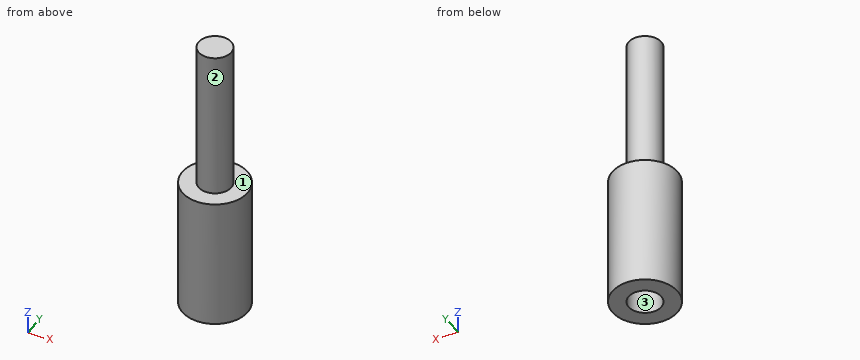
Autodesk Inventor part; units mm, degrees
ref_plane "YZ Plane" through (0, 0, 0) normal (1, 0, 0) x (0, 1, 0)
ref_plane "XZ Plane" through (0, 0, 0) normal (0, 1, 0) x (-1, 0, 0)
ref_plane "XY Plane" through (0, 0, 0) normal (0, 0, 1) x (1, 0, 0)
sketch "Sketch1" plane through (0, 0, 0) normal (0, 0, 1) x (1, 0, 0)
  circle A0 centre (19, -27.5) radius 3
  circle A1 centre (19, -27.5) radius 6
  point P0 (0, 0)
  dimension "d0" = 12
extrude "Extrusion1" add sketch "Sketch1" along normal blind 24.2875
sketch "Sketch2" plane through (19, -27.5, 24.2875) normal (0, 0, 1) x (1, 0, 0)
  circle A0 centre (0, 0) radius 3
  point P0 (-19, 27.5)
  dimension "d3" = 6
extrude "Extrusion2" add sketch "Sketch2" along normal blind 27.4625
sketch "Sketch3" plane through (19, -27.5, 24.2875) normal (0, 0, -1) x (-1, 0, 0)
  circle A0 centre (0, 0) radius 3
  point P0 (19, 27.5)
extrude "Extrusion3" add sketch "Sketch3" along normal blind 10
properties part number "fuckup fixer"
Source: CAD feature listing. Evaluate the final solid. Frame: model axes, mm. Face numbers are marked on the shaded views. Round coordinates to 2 decimals unless told otherwise and drop trailing zeros. Loops run counter-clockwise (first coordinate to the right, second up) from the corner with the lowest first, then second, coordinate; pieces in that order, holes last. Notation, with made-up numbers: M 25,27.5 L 51,27.5 A26 ccw 51,53.5 Z; hole C -14.75,-22 d1. An arc over 180 degrees is marked long. Answer as CSV lines item,"result".
Q1. Cut plane D-D (z = 28.5). Return the cut outline in (x, y).
Verdict:
outline,"C 19,-27.5 d6"
Q2. Cut plane C-C (z = 6). Return the cut outline in (x, y), plus the area to 3 significant figures.
Verdict:
outline,"C 19,-27.5 d12; hole C 19,-27.5 d6"
area,"84.8 mm^2"
Q3. Contact query for flat-ended pins moving along their axis: pin 1 (1 mm diameter, centred on y = -30.5, z = 30.5, fed in from +X); pin 2 (3 mm diameter, centred on y = -24.5, z = 15, fed in from -X); pin 3 (6.5 mm diameter, centred on x = 20, y = -27.5, fed in from -Z); pin 4 (2 mm diameter, centred on y = -23, z = 6, fed in from -X). Output: stop coordinate, or through.
Verdict:
pin 1,"stops at x = 20.66"
pin 2,"stops at x = 13.19"
pin 3,"stops at z = 0"
pin 4,"stops at x = 14.13"
Q4. Cut plane B-B (x = 19). Return the cut outline in (y, z).
Verdict:
outline,"M -33.5,0 L -30.5,0 L -30.5,14.29 L -24.5,14.29 L -24.5,0 L -21.5,0 L -21.5,24.29 L -24.5,24.29 L -24.5,51.75 L -30.5,51.75 L -30.5,24.29 L -33.5,24.29 Z"
Q5. Pull-direction query (Y, two-part tool) for the marked faces 1, 2 and 3; classes: +Y half, -Y half, draft (parallel to the pull), parting line (faces both ways), or undercut.
Verdict:
face 1,"draft"
face 2,"parting line"
face 3,"undercut"
Q6. Line query: line 1 along Y through (x, z) = (19, 5.75); line 2 along Z through (x, y) = (20, -28.25); line 3 along Z through (x, y) = (23.5, -26.5). Output: solid intervals per line, ascending.
Verdict:
line 1,"y = -33.5 to -30.5, -24.5 to -21.5"
line 2,"z = 14.29 to 51.75"
line 3,"z = 0 to 24.29"
Q7. Cut plane A-A (y = -27.5). Return the cut outline in (x, z).
Verdict:
outline,"M 13,0 L 16,0 L 16,14.29 L 22,14.29 L 22,0 L 25,0 L 25,24.29 L 22,24.29 L 22,51.75 L 16,51.75 L 16,24.29 L 13,24.29 Z"
